Could you check a few things on this model? Use its own coordinates, in mm. Face numbers are marked on the shaded views. A direction names the side the tool comes from. Round coordinates to 2 decimals unless told otherwise and drop trailing zeros. Loops run counter-clockwise (first coordinate to the right, second up) from the corner with the lowest first, then second, coordinate; pieces in that order, holes last.
Autodesk Inventor part; units mm, degrees
ref_plane "Plano de trabajo1" through (0, 0, 35) normal (0, 0, 1) x (1, 0, 0)
ref_plane "YZ Plane" through (0, 0, 0) normal (1, 0, 0) x (0, 1, 0)
ref_plane "XZ Plane" through (0, 0, 0) normal (0, 1, 0) x (-1, 0, 0)
sketch "Boceto1" plane through (0, 0, 0) normal (0, 0, 1) x (1, 0, 0)
  line L0 (-52.7575, 20.0575) -> (-32.756, 0)
  line L1 (-32.756, 0) -> (0, 0)
  line L2 (-52.7575, 20.0575) -> (-50.2826, 22.5323)
  line L3 (-52.7575, 20.0575) -> (-49.2575, 20.0575) construction
  line L4 (-50.2826, 22.5323) -> (-31.3034, 3.5)
  line L5 (-31.3034, 3.5) -> (0, 3.5)
  line L6 (0, 0) -> (0, -9.9685) construction
  line L7 (52.7575, 20.0575) -> (32.756, 0)
  line L8 (32.756, 0) -> (0, 0)
  line L9 (52.7575, 20.0575) -> (50.2826, 22.5323)
  line L10 (50.2826, 22.5323) -> (31.3034, 3.5)
  line L11 (31.3034, 3.5) -> (0, 3.5)
  dimension "d0" = 45
  dimension "d1" = 134.92
  dimension "d2" = 3.5
  dimension "d3" = 3.5
  dimension "d4" = 28.326
  dimension "d5" = 32.756
extrude "Extrusión1" add sketch "Boceto1" along normal blind 70
sketch "Boceto2" plane through (0, 0, 70) normal (0, 0, 1) x (1, 0, 0)
  line L0 (-52.7575, 20.0575) -> (-32.756, 0)
  line L1 (-32.756, 0) -> (-48.756, 0)
  line L2 (-48.756, 0) -> (-40.7337, 8)
  line L3 (0, 0) -> (0, -7.1041) construction
  line L4 (52.7575, 20.0575) -> (32.756, 0)
  line L5 (32.756, 0) -> (48.756, 0)
  line L6 (48.756, 0) -> (40.7337, 8)
  point P0 (-47.756, 15.0419)
  dimension "d12" = 16
extrude "Extrusión2" add sketch "Boceto2" against normal blind 3.5
ref_plane "Plano de trabajo1" through (0, 0, 35) normal (0, 0, 1) x (1, 0, 0)
mirror "Simetría1" about plane through (0, 0, 35) normal (0, 0, 1) of "Extrusión2"
sketch "Boceto3" plane through (0, 0, 70) normal (0, 0, 1) x (1, 0, 0)
  circle A0 centre (-39.0001, 3.8002) radius 1.5
  line L0 (-39.0001, 3.8002) -> (-37.7694, 5.0275) construction
  line L1 (-32.756, 0) -> (-40.7337, 8)
  line L2 (0, 0) -> (0, -3.5463) construction
  circle A1 centre (39.0001, 3.8002) radius 1.5
  dimension "d13" = 3
  dimension "d14" = 7.1
  dimension "d15" = 1.738
extrude "Extrusión3" cut sketch "Boceto3" against normal through all
fillet "Empalme1" radius 2 4 edges at (-48.756, 0, 68.25) (48.756, 0, 68.25) (48.756, 0, 1.75) (-48.756, 0, 1.75)
sketch "Boceto4" plane through (0, 0, 0) normal (1, 0, 0) x (0, 1, 0)
  line L0 (6, 62) -> (6, 52) construction
  line L1 (3.5, 59.5) -> (3.5, 54.5)
  line L2 (8.5, 54.5) -> (8.5, 59.5)
  arc A0 (8.5, 59.5) -> (3.5, 59.5) centre (6, 59.5) ccw
  arc A1 (3.5, 54.5) -> (8.5, 54.5) centre (6, 54.5) ccw
  line L3 (3.5, 70) -> (22.5323, 70)
  line L4 (3.5, 0) -> (3.5, 70)
  line L5 (0, 3.5) -> (0, 66.5)
  line L6 (0, 35) -> (-5.0365, 35) construction
  line L7 (3.5, 10.5) -> (3.5, 15.5)
  line L8 (8.5, 15.5) -> (8.5, 10.5)
  arc A2 (3.5, 10.5) -> (8.5, 10.5) centre (6, 10.5) ccw
  arc A3 (8.5, 15.5) -> (3.5, 15.5) centre (6, 15.5) ccw
  point P0 (0, 0)
  point P1 (6, 57)
  point P2 (3.5, 57)
  point P3 (3.5, 15.5)
  point P4 (3.5, 10.5)
  dimension "d19" = 10
  dimension "d20" = 5
  dimension "d21" = 8
extrude "Extrusión4" cut sketch "Boceto4" along normal through all both and the other way through all
properties part number "Soporte_electronica"
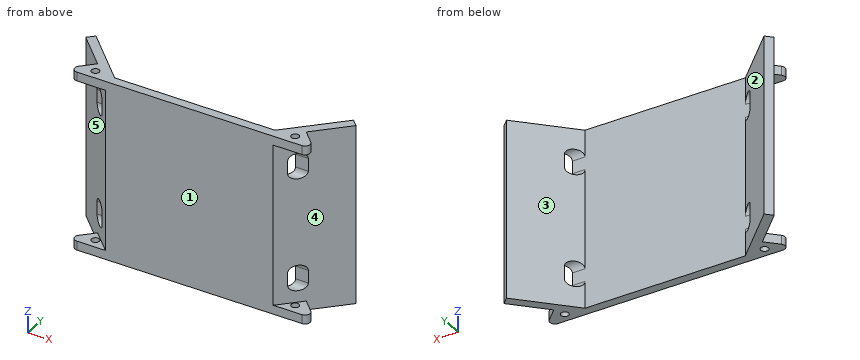
Item 1: We'd pull the mould along Z, two halves only. Please class the marked faces 3, 4 and 5: released by +Z, released by -Z, zero draft, split by the parting line, or undercut.
Results list:
face 3: zero draft
face 4: undercut
face 5: undercut
Item 2: If we section it at D-D, the plane y = 16: Please give me the cut outline in (x, z).
Results list:
outline: (-48.71, 0) - (-43.77, 0) - (-43.77, 70) - (-48.71, 70) - close; (43.77, 0) - (48.71, 0) - (48.71, 70) - (43.77, 70) - close
Item 3: For the marked faces 1 and 2, which set-ups out of +Z, -Z, +X, -X, +Y, -Y let a thin tool reach every point of the face, with its end or its side?
Results list:
face 1: +Z, -Z, +X, -X, -Y
face 2: +Z, -Z, +Y
Item 4: If I drill on line 1 along Z through (x, y) = (-42.5, 3); line 2 along Y through (x, z) = (-30.5, 28); line 3 along X through (y, z) = (17, 8), over which ranges is the centre line in solid material (lowest first)?
Results list:
line 1: z = 0 to 3.5, 66.5 to 70
line 2: y = 0 to 3.5
line 3: x = -49.71 to -44.77, 44.77 to 49.71
Item 5: If we section it at A-A, the plane z = 56.5: Please give me the cut outline in (x, y).
Results list:
outline: (-52.76, 20.06) - (-41.23, 8.5) - (-36.29, 8.5) - (-50.28, 22.53) - close; (-36.25, 3.5) - (-32.76, 0) - (32.76, 0) - (36.25, 3.5) - close; (36.29, 8.5) - (41.23, 8.5) - (52.76, 20.06) - (50.28, 22.53) - close
Item 6: Will these pins go through, and if not, where does the flat tip stop? pin 1 (3.5 mm diameter, centred on x = -39, y = 3.8, fed in from -Z); pin 2 (1.5 mm diameter, centred on x = 18, z = 40.5, fed in from +Y); pin 3 (2.5 mm diameter, centred on x = 38, z = 56.5, fed in from -Y); pin 4 (4 mm diameter, centred on x = 40, z = 12, fed in from -Y).
Results list:
pin 1: stops at z = 0
pin 2: stops at y = 3.5
pin 3: stops at y = 8.5
pin 4: stops at y = 8.45
Item 7: If we section it at B-B, the plane y = 6.75: Count the separate pieces of the cut face and the enclosed holes in it, then the cut area to 3 significant figures.
Results list:
separate pieces: 6
enclosed holes: 0
area: 534 mm2
Item 8: If we section it at C-C, the plane z = 36: Please give me the cut outline in (x, y), then the cut area to 3 significant figures.
Results list:
outline: (-52.76, 20.06) - (-32.76, 0) - (32.76, 0) - (52.76, 20.06) - (50.28, 22.53) - (31.3, 3.5) - (-31.3, 3.5) - (-50.28, 22.53) - close
area: 417 mm2
